The model under review builds one solid part; all positions refer to its coordinate system, in mm. A direction names the side the tool comes from. Coordinates: 2 decimals unless noted, no trailing zeros. Write each loop counter-clockwise with the first axis right and the second up, starting at its lowest first coordinate (ties: lowest second). Pieces come first, ordered by that corner, then holes.
1) Add section A-A, the plane y = 0. Give the number of separate pieces and of enclosed holes in the cut face, then the cut area to 3 significant figures.
2) For line 1 (Y direction, x = 0.8, z = -6); line 2 (X direction, y = -2.5, z = 10.5); line 3 (Z direction, x = 1.2, y = 0), list the stretches that pass through material, from the lowest coordinate up.
3) Machinability: for faces 1 (the flat face through (-3.1, 0, 9)), 2 (the cylindrical face through (0.034, -3.199, -14.715)), 3 (the flat face through (-2.4, 0, -9)), 4 (the flat face through (2.4, 0, -9)), which of the approach directions +Z, -Z, +X, -X, +Y, -Y give a long, thin tool a straight path to every point of the face, cutting with its end or side? Answer none if there is none.
4) Add section D-D, the plane z = -6. State the section outline as (x, y) points.
5) Mouldability with a two-part tool opening along X and no side actions: class faces 5 (the cylindrical face through (5.331, -3.199, 14.715)), 6 (the flat face through (0, 0, 5)), 7 (the flat face through (7.5, 0, 9)), 8 (the flat face through (3.1, 0, 9)) as released by +X, released by -X, zero draft, split by the parting line, or undercut.
6) For P1, Ø0.9, axis at x = 5, y = 0, coming from the -Z side; P2, Ø1.3, axis at x = 0, y = -1.5, coming from the +Z side; P3, Ø3.5, axis at y = -0.5, z = -9.5, coming from the +X side, all flat-tipped, find the tip position at first contact; note any pin that passes through.
7) Add section B-B, the plane z = 11. State the section outline as (x, y) points.
8) Add section C-C, the plane x = 1.25. State the section outline as (y, z) points.
from build123d import *
from build123d.topology import SkipClean

# Parameters (mm, degrees)
SALIENTE_EXTRUIR1_DEPTH    = 2.4
CORTAR_EXTRUIR1_DEPTH      = 16.588778015
CORTAR_EXTRUIR1_DEPTH_BACK = 16.588778015
CROQUIS2_R                 = 1.5
CROQUIS3_R                 = 1.5
SALIENTE_EXTRUIR2_DEPTH    = 7.5
CORTAR_EXTRUIR2_DEPTH      = 3.1
REDONDEO1_R                = 2
REDONDEO2_R                = 1


with BuildPart() as part:
    # Croquis1 → Saliente-Extruir1 (new, symmetric)
    with BuildSketch(Plane(origin=(0, 0, 0), x_dir=(0, 0, -1), z_dir=(1, 0, 0))):
        with BuildLine():
            Line((-14, 3.5), (14, 3.5))
            ThreePointArc((14, 3.5), (14.707106781, 3.207106781), (15, 2.5))
            Line((15, 2.5), (15, -2.5))
            ThreePointArc((15, -2.5), (14.707106781, -3.207106781), (14, -3.5))
            Line((14, -3.5), (-14, -3.5))
            ThreePointArc((-14, -3.5), (-14.707106781, -3.207106781), (-15, -2.5))
            Line((-15, -2.5), (-15, 2.5))
            ThreePointArc((-15, 2.5), (-14.707106781, 3.207106781), (-14, 3.5))
        make_face()
    extrude(amount=SALIENTE_EXTRUIR1_DEPTH, both=True)

    # Croquis2 → Cortar-Extruir1 (cut, two sides: drawn at the far end of the back side and taken through both)
    with BuildSketch(Plane(origin=(0, 0, 0), x_dir=(0, 0, -1), z_dir=(1, 0, 0)).offset(-CORTAR_EXTRUIR1_DEPTH_BACK)):
        with Locations((-11, 0)):
            Circle(CROQUIS2_R)
        with Locations((6, 0)):
            Circle(CROQUIS2_R)
    extrude(amount=CORTAR_EXTRUIR1_DEPTH + CORTAR_EXTRUIR1_DEPTH_BACK, mode=Mode.SUBTRACT)

    # Croquis3 → Saliente-Extruir2 (add, symmetric)
    with SkipClean():  # the faces are left unmerged after this step: merging them gives an invalid solid
        with BuildSketch(Plane(origin=(0, 0, 0), x_dir=(0, 0, -1), z_dir=(1, 0, 0))):
            with BuildLine():
                Line((-15, 2.5), (-15, -2.5))
                ThreePointArc((-15, -2.5), (-14.707106781, -3.207106781), (-14, -3.5))
                Line((-14, -3.5), (0, -3.5))
                Line((0, -3.5), (0, 3.5))
                Line((0, 3.5), (-14, 3.5))
                ThreePointArc((-14, 3.5), (-14.707106781, 3.207106781), (-15, 2.5))
            make_face()
            with Locations((-11, 0)):
                Circle(CROQUIS3_R, mode=Mode.SUBTRACT)
        extrude(amount=SALIENTE_EXTRUIR2_DEPTH, both=True)
    add(part.part.scale(1), mode=Mode.REPLACE)  # the faces are merged on a copy

    # Croquis4 → Cortar-Extruir2 (cut, symmetric)
    with BuildSketch(Plane(origin=(0, 0, 0), x_dir=(0, 0, -1), z_dir=(1, 0, 0))):
        with BuildLine():
            Line((-14, 3.5), (-5, 3.5))
            Line((-5, 3.5), (-5, -3.5))
            Line((-5, -3.5), (-14, -3.5))
            ThreePointArc((-14, -3.5), (-14.707106781, -3.207106781), (-15, -2.5))
            Line((-15, -2.5), (-15, 2.5))
            ThreePointArc((-15, 2.5), (-14.707106781, 3.207106781), (-14, 3.5))
        make_face()
    extrude(amount=CORTAR_EXTRUIR2_DEPTH, both=True, mode=Mode.SUBTRACT)

    # Redondeo1
    redondeo1_edges = [part.edges().sort_by_distance(p)[0] for p in [
        (-2.4, 0, 0),
        (2.4, 0, 0),
        (-7.5, 0, 0),
        (7.5, 0, 0),
    ]]
    fillet(redondeo1_edges, radius=REDONDEO1_R)

    # Redondeo2
    redondeo2_edges = [part.edges().sort_by_distance(p)[0] for p in [
        (3.1, 0, 5),
        (-3.1, 0, 5),
    ]]
    fillet(redondeo2_edges, radius=REDONDEO2_R)


solid = part.part
Geometry results:
1. separate pieces: 4
1. enclosed holes: 0
1. area: 195 mm2
2. line 1: y = -3.5 to -1.5, 1.5 to 3.5
2. line 2: x = -7.5 to -3.1, 3.1 to 7.5
2. line 3: z = -15 to -7.5, -4.5 to 5
3. face 1: +Z, +Y, -Y
3. face 2: -Z, +X, -X, -Y
3. face 3: -Z, -X, +Y, -Y
3. face 4: -Z, +X, +Y, -Y
4. outline: (-2.4, -3.5) - (2.4, -3.5) - (2.4, -1.5) - (-2.4, -1.5) - close; (-2.4, 1.5) - (2.4, 1.5) - (2.4, 3.5) - (-2.4, 3.5) - close
5. face 5: zero draft
5. face 6: undercut
5. face 7: released by +X
5. face 8: undercut
6. P1: stops at z = 0
6. P2: stops at z = 5
6. P3: stops at x = 2.4
7. outline: (-7.5, -3.5) - (-3.1, -3.5) - (-3.1, -1.5) - (-7.5, -1.5) - close; (-7.5, 1.5) - (-3.1, 1.5) - (-3.1, 3.5) - (-7.5, 3.5) - close; (3.1, -3.5) - (7.5, -3.5) - (7.5, -1.5) - (3.1, -1.5) - close; (3.1, 1.5) - (7.5, 1.5) - (7.5, 3.5) - (3.1, 3.5) - close
8. outline: (-3.5, -14) arc R1 ccw to (-2.5, -15) - (2.5, -15) arc R1 ccw to (3.5, -14) - (3.5, 5) - (-3.5, 5) - close; hole circle Ø3 at (0, -6)
